```python
from build123d import *

# Parameters (mm, degrees)
F0_W     = 25
F0_H     = 1
F0_W_2   = 0.2
F0_H_2   = 0.2
F1_DEPTH = 4


with BuildPart() as f1:
    # F0 (on Top) → F1 (new body)
    with BuildSketch(Plane.XY):
        Polygon((70, 90), (0, 90), (-70, 90), (-80, 80), (-80, 30), (-70, 20), (-45, 20), (-40, 15), (-40, 0), (-40, -15), (-45, -20), (-70, -20), (-80, -30), (-80, -80), (-70, -90), (0, -90), (70, -90), (80, -80), (80, -30), (70, -20), (45, -20), (40, -15), (40, 0), (40, 15), (45, 20), (70, 20), (80, 30), (80, 80), align=None)
        with Locations((-59.5, -78)):
            Rectangle(F0_W, F0_H, mode=Mode.SUBTRACT)
        with Locations((-37, -59.5)):
            Rectangle(F0_W_2, F0_H_2, mode=Mode.SUBTRACT)
        with Locations((-23, -59.5)):
            Rectangle(F0_W_2, F0_H_2, mode=Mode.SUBTRACT)
        with Locations((-59.5, -32)):
            Rectangle(F0_W, F0_H, mode=Mode.SUBTRACT)
        Polygon((12.5, -78.5), (0, -78.5), (-12.5, -78.5), (-12.5, -77.5), (0, -77.5), (12.5, -77.5), align=None, mode=Mode.SUBTRACT)
        with Locations((23, -59.5)):
            Rectangle(F0_W_2, F0_H_2, mode=Mode.SUBTRACT)
        with Locations((37, -59.5)):
            Rectangle(F0_W_2, F0_H_2, mode=Mode.SUBTRACT)
        with Locations((59.5, -78)):
            Rectangle(F0_W, F0_H, mode=Mode.SUBTRACT)
        Polygon((12.5, -32.5), (0, -32.5), (-12.5, -32.5), (-12.5, -31.5), (0, -31.5), (12.5, -31.5), align=None, mode=Mode.SUBTRACT)
        with Locations((59.5, -32)):
            Rectangle(F0_W, F0_H, mode=Mode.SUBTRACT)
        with Locations((-59.5, 32)):
            Rectangle(F0_W, F0_H, mode=Mode.SUBTRACT)
        with Locations((-59.5, 78)):
            Rectangle(F0_W, F0_H, mode=Mode.SUBTRACT)
        with Locations((-37, 59.5)):
            Rectangle(F0_W_2, F0_H_2, mode=Mode.SUBTRACT)
        with Locations((-23, 59.5)):
            Rectangle(F0_W_2, F0_H_2, mode=Mode.SUBTRACT)
        Polygon((12.5, 32.5), (12.5, 31.5), (0, 31.5), (-12.5, 31.5), (-12.5, 32.5), (0, 32.5), align=None, mode=Mode.SUBTRACT)
        with Locations((59.5, 32)):
            Rectangle(F0_W, F0_H, mode=Mode.SUBTRACT)
        with Locations((23, 59.5)):
            Rectangle(F0_W_2, F0_H_2, mode=Mode.SUBTRACT)
        with Locations((37, 59.5)):
            Rectangle(F0_W_2, F0_H_2, mode=Mode.SUBTRACT)
        Polygon((-12.5, 78.5), (0, 78.5), (12.5, 78.5), (12.5, 77.5), (0, 77.5), (-12.5, 77.5), align=None, mode=Mode.SUBTRACT)
        with Locations((59.5, 78)):
            Rectangle(F0_W, F0_H, mode=Mode.SUBTRACT)
    extrude(amount=F1_DEPTH)


solid = f1.part
```
CAD build for the part. Positions are in the model's coordinates, mm. A direction names the side the tool comes from. Round coordinates to 2 decimals unless told otherwise and drop trailing zeros. Order: outer loops, then holes, each group sorted by start corner. A loop starts at its lowest first (then second) coordinate and runs counter-clockwise, first axis right, second up. Notation, with made-up numbers: (-29.75, 3.5) - (29.25, 3.5) arc R32 cw to (29.25, 33.5) - close; hole circle Ø1 at (42, 14). An arc over 180 degrees is marked (long way). Answer in a Markdown table with one row per item. Add a question column.
(1) Probe L1, parallel to Y at x = -5, z = 0.4; L2, parallel to Y at x = -48, z = 1.65; L3, parallel to X at y = 14, z = 0.85. List the from-to ranges inside material, lowest first. Write a range as [from, to].
(2) Band-saw the part on D-D on y = -7. List the corners of the cut face in (x, z).
(3) 3-axis set-ups, long thin cutter, end or side, ignore diameter. For faces 4 (the face through (42, 17, 2)), 5 (the face through (59, -78.5, 2)), 6 (the face through (-57, -20, 2)), 7 (the face through (75, 85, 2)): which of +Z, -Z, +X, -X, +Y, -Y reach the whole face in a straight line?
(4) Band-saw the part on C-C on z = 1. Count the separate pieces of the cut face and the enclosed holes in it, and give its area (3 significant figures).
(5) Drop a flat-ended pin along its axis: pin 1 Ø6 at (x, y) = (43.5, 33.5) entering from -Z. Give the stop position or say it passes through.
(6) Band-saw the part on A-A on x = -50. List the corners of the cut face in (y, z), and give its area (3 significant figures).
(7) Band-saw the part on B-B on x = 6. List the corners of the cut face in (y, z).
(8) Mould opens along X. For faces 1 (the face through (0, 31.5, 2)), 2 (the face through (58, -20, 2)), 3 (the face through (75, 25, 2)) say: +X half, -X half, draft (parallel to the pull), parting line (faces both ways), or undercut.
Data:
| question | item | result |
|---|---|---|
| 1 | L1 | y = [-90, -78.5], [-77.5, -32.5], [-31.5, 31.5], [32.5, 77.5], [78.5, 90] |
| 1 | L2 | y = [-90, -78.5], [-77.5, -32.5], [-31.5, -20], [20, 31.5], [32.5, 77.5], [78.5, 90] |
| 1 | L3 | x = [-40, 40] |
| 2 | outline | (-40, 0) - (40, 0) - (40, 4) - (-40, 4) - close |
| 3 | face 4 | +Z, -Z, +X |
| 3 | face 5 | +Z, -Z |
| 3 | face 6 | +Z, -Z, -X |
| 3 | face 7 | +Z, -Z, +X, +Y |
| 4 | separate pieces | 1 |
| 4 | enclosed holes | 20 |
| 4 | area | 24,900 mm^2 |
| 5 | pin 1 | stops at z = 0 |
| 6 | outline | (-90, 0) - (-78.5, 0) - (-78.5, 4) - (-90, 4) - close; (-77.5, 0) - (-32.5, 0) - (-32.5, 4) - (-77.5, 4) - close; (-31.5, 0) - (-20, 0) - (-20, 4) - (-31.5, 4) - close; (20, 0) - (31.5, 0) - (31.5, 4) - (20, 4) - close; (32.5, 0) - (77.5, 0) - (77.5, 4) - (32.5, 4) - close; (78.5, 0) - (90, 0) - (90, 4) - (78.5, 4) - close |
| 6 | area | 544 mm^2 |
| 7 | outline | (-90, 0) - (-78.5, 0) - (-78.5, 4) - (-90, 4) - close; (-77.5, 0) - (-32.5, 0) - (-32.5, 4) - (-77.5, 4) - close; (-31.5, 0) - (31.5, 0) - (31.5, 4) - (-31.5, 4) - close; (32.5, 0) - (77.5, 0) - (77.5, 4) - (32.5, 4) - close; (78.5, 0) - (90, 0) - (90, 4) - (78.5, 4) - close |
| 8 | face 1 | undercut |
| 8 | face 2 | draft |
| 8 | face 3 | +X half |
